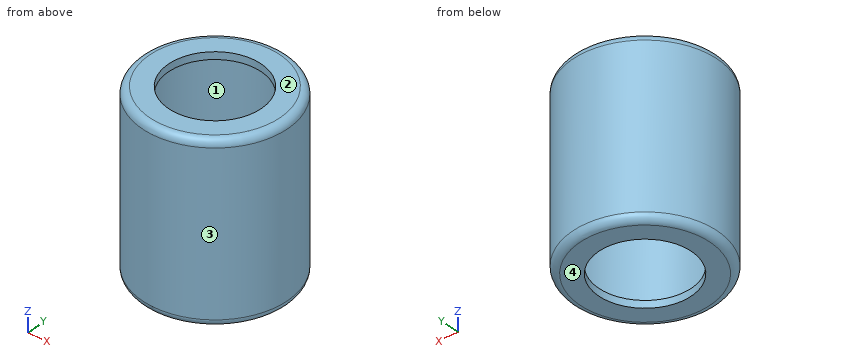
from build123d import *

# Parameters (mm, degrees)
FILLET_1_R = 0.3
FILLET_2_R = 0.5
FILLET_3_R = 0.5


with BuildPart() as part:
    # 草图1 → 旋转1 (revolve)
    with BuildSketch(Plane(origin=(0, 0, 0), x_dir=(1, 0, 0), z_dir=(0, 1, 0))):
        Polygon((3.2, -6), (5, -6), (5, 6), (3.2, 6), (3.2, 5.5), (4.5, 5.5), (4.5, -5.5), (3.2, -5.5), align=None)
    revolve(axis=Axis((0, 0, 32.403310218), (0, 0, -1)))

    # 圆角1
    fillet_1_edges = [part.edges().sort_by_distance(p)[0] for p in [
        (-4.5, 0, 5.5),
        (-4.5, 0, -5.5),
    ]]
    fillet(fillet_1_edges, radius=FILLET_1_R)

    # 圆角2
    fillet_2_edges = [part.edges().sort_by_distance(p)[0] for p in [
        (-5, 0, 6),
    ]]
    fillet(fillet_2_edges, radius=FILLET_2_R)

    # 圆角3
    fillet_3_edges = [part.edges().sort_by_distance(p)[0] for p in [
        (-5, 0, -6),
    ]]
    fillet(fillet_3_edges, radius=FILLET_3_R)


solid = part.part
For this review, take the finished solid that the model builds, in its own axes (mm). Face numbers are marked on the shaded views. Round coordinates to 2 decimals unless told otherwise and drop trailing zeros. Loops run counter-clockwise (first coordinate to the right, second up) from the corner with the lowest first, then second, coordinate; pieces in that order, holes last. Notation, with made-up numbers: (-16.5, 9.5) - (-5.5, 9.5) arc R17 ccw to (-5.5, 21.5) - close; hole circle Ø5 at (52, 49). An arc over 180 degrees is marked (long way). Use one line per item in the form item = value.
1) Clearance check with flat-ended pins moving along their axes: P1, Ø3, axis at x = 4, z = -3.5, coming from the -Y side; P2, Ø5, axis at x = 0, y = 0, coming from the +Z side; P3, Ø2, axis at y = -2.5, z = 0.5, coming from the +X side. State where each tip first meets the part, or that it passes through.
Solutions:
P1 = -4.33
P2 = through
P3 = 4.77
2) Wall thickness on probe 1 along Z at (x, y) = (3.25, -0.5); probe 2 along Y at (x, z) = (0, 2): over which ranges is each line inside the solid? List them lowest first.
Solutions:
probe_1 = -6 to -5.5, 5.5 to 6
probe_2 = -5 to -4.5, 4.5 to 5
3) We need section C-C on z = 2.25. Write out the cut boundary in (x, y), then the cut area to 3 significant figures.
Solutions:
outline = circle Ø10 at (0, 0); hole circle Ø9 at (0, 0)
area = 14.9 mm2
4) We need section A-A on y = 0. Write out the cut boundary in (x, z), then the cut area to 3 significant figures.
Solutions:
outline = (-5, -5.5) arc R0.5 ccw to (-4.5, -6) - (-3.2, -6) - (-3.2, -5.5) - (-4.2, -5.5) arc R0.3 cw to (-4.5, -5.2) - (-4.5, 5.2) arc R0.3 cw to (-4.2, 5.5) - (-3.2, 5.5) - (-3.2, 6) - (-4.5, 6) arc R0.5 ccw to (-5, 5.5) - close; (3.2, -6) - (4.5, -6) arc R0.5 ccw to (5, -5.5) - (5, 5.5) arc R0.5 ccw to (4.5, 6) - (3.2, 6) - (3.2, 5.5) - (4.2, 5.5) arc R0.3 cw to (4.5, 5.2) - (4.5, -5.2) arc R0.3 cw to (4.2, -5.5) - (3.2, -5.5) - close
area = 14.5 mm2
5) Mouldability with a two-part tool opening along Z and no side actions: class the marked faces 1, 2, 3 and 4 as pulls with the +Z half, pulls with the -Z half, needs draft (parallel to the pull), parting line crosses it, or undercut.
Solutions:
face_1 = undercut
face_2 = pulls with the +Z half
face_3 = needs draft
face_4 = pulls with the -Z half
